Study the drawing (mm; zero at the part's minimum x, y, z) and answer. Give positions to 0.01 mm unless a question says otherwise; leave off trailing zeros. Write each loop counter-clockwise with the first axis right and the second up, starting at its lowest first coordinate (ties: lowest second). Pieces come first, ordered by that corner, then holes. Notation, with made-up numbers: (35.5, 8.25) - (44.5, 8.25) arc R16 cw to (44.5, 38.25) - close; hole circle Ø9 at (87, 69.5). An arc over 180 degrees is marked (long way). Return JSON: item names as keys, results as strings.
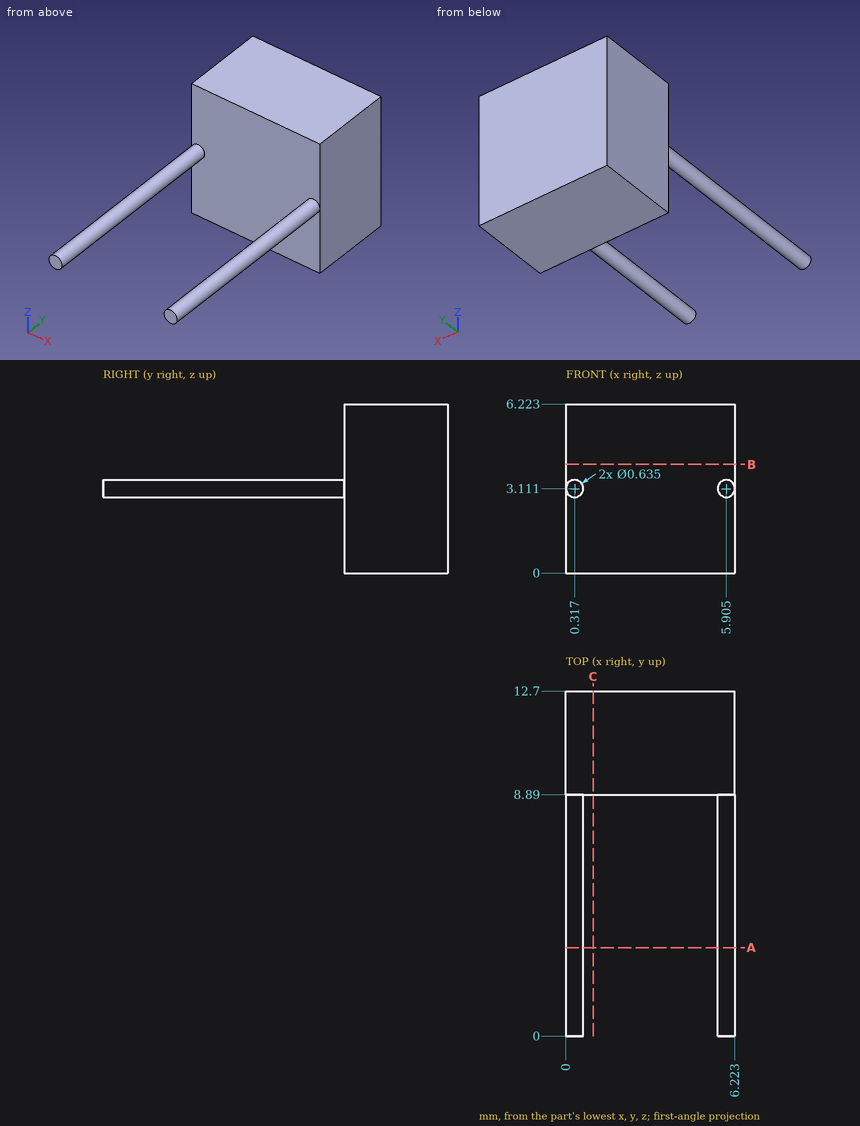
Item 1: A flat-ended cylindrical pin translates along its axis: P1, Ø1, axis at x = 4, z = 2, coming from the -Y side. Find the tip coordinate at first contact, or state that the pin passes through.
Answer below:
{"P1": "stops at y = 8.89"}
Item 2: Consider L1, parallel to Y at x = 0.5, z = 1.75; L2, parallel to X at y = 6.5, z = 3.25 (1 decimal). Determine where each line is inside the solid, lowest interval first.
Answer below:
{"L1": "y = 8.89 to 12.7", "L2": "x = 0 to 0.6, 5.6 to 6.2"}
Item 3: A cutting plane is placed at C-C on x = 1. Determine the outline of the cut face in (y, z).
Answer below:
{"outline": "(8.89, 0) - (12.7, 0) - (12.7, 6.22) - (8.89, 6.22) - close"}
Item 4: A cutting plane is placed at A-A on y = 3.25. Determine the outline of the cut face in (x, z) (1 decimal).
Answer below:
{"outline": "circle Ø0.6 at (0.3, 3.1); circle Ø0.6 at (5.9, 3.1)"}
Item 5: A cutting plane is placed at B-B on z = 4. Determine the outline of the cut face in (x, y), then the cut area to 3 significant figures.
Answer below:
{"outline": "(0, 8.89) - (6.22, 8.89) - (6.22, 12.7) - (0, 12.7) - close", "area": "23.7 mm²"}
